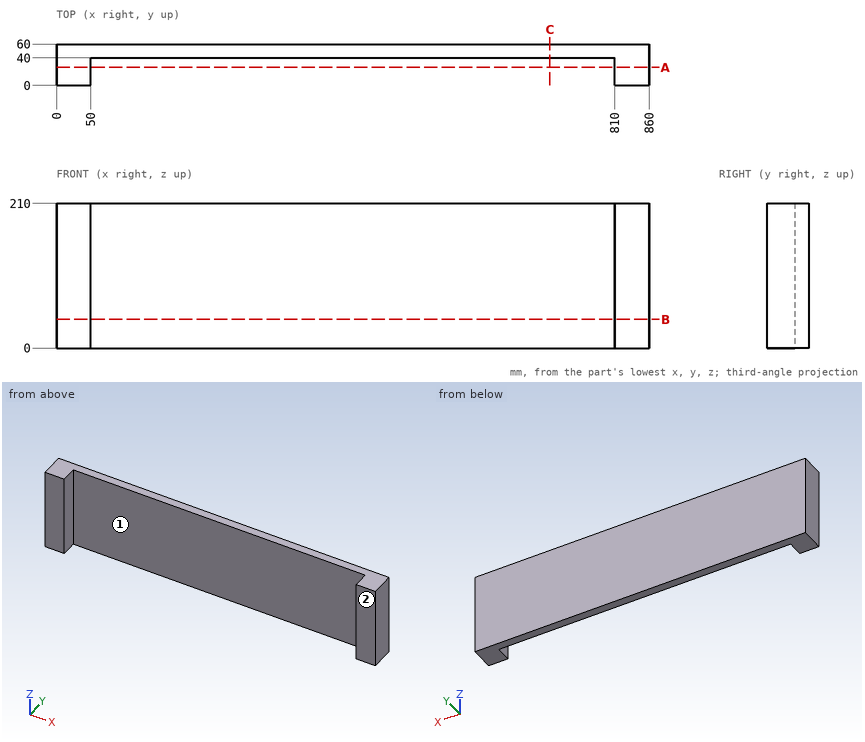
Can you work these out from the drawing? Everything is in mm from the part's minimum corner. Give positions to 0.01 mm unless a question says otherwise; leave off trailing zeros. Loops run counter-clockwise (first coordinate to the right, second up) from the corner with the lowest first, then second, coordinate; pieces in that order, holes last. Notation, with made-up numbers: (69, 43) -> (119, 43) arc R18 cw to (119, 65) -> close; hole circle Ø11 at (22.25, -4). An arc over 180 degrees is marked (long way). Write item = value, one per line.
1) Will this pin go through, and if not, where does the flat tip stop? pin 1 (3 mm diameter, centred on x = 588.5, z = 101, fed in from -Y).
Check result:
pin_1 = 40
2) Suppose I cut it at C-C on x = 716. Write out the boundary of the cut face in (y, z), then the cut area to 3 significant figures.
Check result:
outline = (40, 0) -> (60, 0) -> (60, 210) -> (40, 210) -> close
area = 4,200 mm2
3) Suppose I cut it at B-B on z = 41.5. Write out the boundary of the cut face in (x, y), then the cut area to 3 significant figures.
Check result:
outline = (0, 0) -> (50, 0) -> (50, 40) -> (810, 40) -> (810, 0) -> (860, 0) -> (860, 60) -> (0, 60) -> close
area = 21,200 mm2
4) Thinking about a two-plate mould opening in X: for the marked faces 1 and 2, which applies, released by +X, released by -X, zero draft, split by the parting line, or undercut?
Check result:
face_1 = undercut
face_2 = zero draft
5) Suppose I cut it at A-A on y = 26. Write out the boundary of the cut face in (x, z), then the cut area to 3 significant figures.
Check result:
outline = (0, 0) -> (50, 0) -> (50, 210) -> (0, 210) -> close; (810, 0) -> (860, 0) -> (860, 210) -> (810, 210) -> close
area = 21,000 mm2
6) I need wall thicknesses on L1, parallel to X at y = 31, z = 192; L2, parallel to Y at x = 693, z = 80. Which ranges of each line are inside material? Lowest first, please. Write a range as from..to.
Check result:
L1 = 0..50, 810..860
L2 = 40..60
